Build history of the part. All positions in model axes, mm. Face numbers are marked on the shaded views. A direction names the side the tool comes from. Coordinates: 2 decimals unless noted, no trailing zeros. Order: outer loops, then holes, each group sorted by start corner. A loop starts at its lowest first (then second) coordinate and runs counter-clockwise, first axis right, second up. Notation, with made-up numbers: M 86,-35 L 118,-35 A35 cw 118,1 Z; hole C 27,8.5 d3. An arc over 180 degrees is marked long. Write item = value, one per line. Start each with the question number.
Q1. Pull direction X, two halves, no side cores. Call the marked faces 1, 2 and 3: released by +X, released by -X, zero draft, split by the parting line, or undercut.
Q2. Pin check, flat tips, straight feed: P1, Ø0.9, axis at y = -18.5, z = 9.5, coming from the +X side; P2, Ø2, axis at x = 0.5, y = -22.5, coming from the +Z side; P3, Ø0.5, axis at y = -9, z = 8.5, coming from the +X side; P4, Ø0.8, axis at x = -11, z = 8.5, coming from the +Y side. Stop position of each tip, or through.
Q3. Band-saw the part on D-D on x = -18. Write the cut outline in (y, z), plus the area to 3 significant figures.
Q4. 3-axis set-ups, long thin cutter, end or side, ignore diameter. For the marked faces 4, 5 and 6: which of +Z, -Z, +X, -X, +Y, -Y reach the whole face in a straight line?
Q5. Drill centre lines: probe 1 along X at (y, z) = (-17, 15); probe 2 along X at (y, z) = (-18.25, 9); probe 3 along X at (y, z) = (-24.25, 9). Where is each one in solid material? Low to high.
Q6. Band-saw the part on B-B on z = 14.75. Write the cut outline in (x, y), plus the area to 3 significant figures.
Q7. Band-saw the part on A-A on z = 10. Write the cut outline in (x, y), plus the area to 3 significant figures.
Q8. Band-saw the part on C-C on z = 7. State how many separate pieces and enclosed holes the cut face has, plus the area to 3 significant figures.
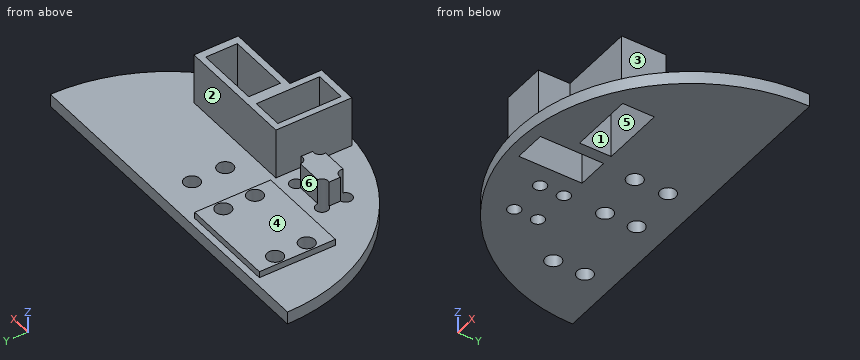
```python
from build123d import *

# Parameters (mm, degrees)
SKETCH009_W      = 5
SKETCH009_H      = 10
SKETCH009_W_2    = 10
SKETCH009_H_2    = 5
EXTRUDE008_DEPTH = 10
SKETCH008_R      = 1
EXTRUDE007_DEPTH = 6
SKETCH007_R      = 1.25
EXTRUDE006_DEPTH = 3
SKETCH004_R      = 1.25
EXTRUDE005_DEPTH = 3
SKETCH005_W      = 6.5
SKETCH005_H      = 4
EXTRUDE004_DEPTH = 4
SKETCH006_W      = 12
SKETCH006_H      = 7
SKETCH006_W_2    = 7
SKETCH006_H_2    = 12
EXTRUDE003_DEPTH = 8
SKETCH003_W      = 15
SKETCH003_H      = 12
EXTRUDE002_DEPTH = 1
EXTRUDE001_DEPTH = 6
EXTRUDE_DEPTH    = 8


with BuildPart() as usb_cuts:
    # Sketch009 → Extrude008 (new body)
    with BuildSketch(Plane.XY.offset(16)):
        with Locations((0, -20.5)):
            Rectangle(SKETCH009_W, SKETCH009_H)
        with Locations((9.25, -18)):
            Rectangle(SKETCH009_W_2, SKETCH009_H_2)
    extrude(amount=-EXTRUDE008_DEPTH)


with BuildPart() as reset_leads:
    # Sketch008 → Extrude007 (new body)
    with BuildSketch(Plane.XY.offset(12)):
        with Locations((-12, -16)):
            Circle(SKETCH008_R)
        with Locations((-6, -19.75)):
            Circle(SKETCH008_R)
        with Locations((-6, -16)):
            Circle(SKETCH008_R)
        with Locations((-12, -19.75)):
            Circle(SKETCH008_R)
    extrude(amount=-EXTRUDE007_DEPTH)


with BuildPart() as momentary_leads:
    # Sketch007 → Extrude006 (new body)
    with BuildSketch(Plane.XY.offset(9)):
        with Locations((-18, -9.5)):
            Circle(SKETCH007_R)
        with Locations((-18, -4.5)):
            Circle(SKETCH007_R)
        with Locations((-6, -9.5)):
            Circle(SKETCH007_R)
        with Locations((-6, -4.5)):
            Circle(SKETCH007_R)
    extrude(amount=-EXTRUDE006_DEPTH)


with BuildPart() as obj1:
    # Sketch004 → Extrude005 (new body)
    with BuildSketch(Plane.XY.offset(8)):
        with Locations((2, -10.25)):
            Circle(SKETCH004_R)
        with Locations((2, -5)):
            Circle(SKETCH004_R)
    extrude(amount=-EXTRUDE005_DEPTH)


with BuildPart() as obj2:
    # Sketch005 → Extrude004 (new body)
    with BuildSketch(Plane.XY.offset(8)):
        with Locations((-9, -18)):
            Rectangle(SKETCH005_W, SKETCH005_H)
    extrude(amount=EXTRUDE004_DEPTH)


with BuildPart() as usb_ports001:
    # Sketch006 → Extrude003 (new body)
    with BuildSketch(Plane.XY.offset(8)):
        with Locations((9.5, -18)):
            Rectangle(SKETCH006_W, SKETCH006_H)
        with Locations((0, -20.5)):
            Rectangle(SKETCH006_W_2, SKETCH006_H_2)
    extrude(amount=EXTRUDE003_DEPTH)


with BuildPart() as momentary_button:
    # Sketch003 → Extrude002 (new body)
    with BuildSketch(Plane.XY.offset(8)):
        with Locations((-12, -7)):
            Rectangle(SKETCH003_W, SKETCH003_H)
    extrude(amount=EXTRUDE002_DEPTH)


with BuildPart() as body_cut:
    # Sketch002 → Extrude001 (new body)
    with BuildSketch(Plane.XY):
        with BuildLine():
            ThreePointArc((-27.5, 0), (0, -27.5), (27.5, 0))
            Line((-27.5, 0), (27.5, 0))
        make_face()
    extrude(amount=EXTRUDE001_DEPTH)


with BuildPart() as cut004:
    # Sketch001 → Extrude (new body)
    with BuildSketch(Plane.XY):
        with BuildLine():
            ThreePointArc((-27.5, 0), (0, -27.5), (27.5, 0))
            Line((-27.5, 0), (27.5, 0))
        make_face()
    extrude(amount=EXTRUDE_DEPTH)

    # Cut: cut Body Cut
    add(body_cut.part, mode=Mode.SUBTRACT)

    # Fusion: union Momentary Button
    add(momentary_button.part)

    # Fusion001: union USB Ports001
    add(usb_ports001.part)

    # Fusion002: union obj2
    add(obj2.part)

    # Cut001: cut obj1
    add(obj1.part, mode=Mode.SUBTRACT)

    # Cut002: cut momentary Leads
    add(momentary_leads.part, mode=Mode.SUBTRACT)

    # Cut003: cut Reset Leads
    add(reset_leads.part, mode=Mode.SUBTRACT)

    # Cut004: cut USB Cuts
    add(usb_cuts.part, mode=Mode.SUBTRACT)


solid = cut004.part
```
Recorded:
q1.face_1 = undercut
q1.face_2 = zero draft
q1.face_3 = released by +X
q2.P1 = 15.5
q2.P2 = through
q2.P3 = -4.5
q2.P4 = -1
q3.outline = M -20.79,6 L -10.75,6 L -10.75,9 L -13,9 L -13,8 L -20.79,8 Z; M -8.25,6 L -5.75,6 L -5.75,9 L -8.25,9 Z; M -3.25,6 L 0,6 L 0,8 L -1,8 L -1,9 L -3.25,9 Z
q3.area = 38.6 mm2
q4.face_4 = +Z, +X, -X, +Y
q4.face_5 = +Z, -Z
q4.face_6 = +Z, -X
q5.probe_1 = -3.5 to -2.5, 2.5 to 4.25, 14.25 to 15.5
q5.probe_2 = -12.25 to -5.75, -3.5 to -2.5, 2.5 to 4.25, 14.25 to 15.5
q5.probe_3 = -3.5 to -2.5, 2.5 to 3.5
q6.outline = M -3.5,-26.5 L 3.5,-26.5 L 3.5,-21.5 L 15.5,-21.5 L 15.5,-14.5 L -3.5,-14.5 Z; hole M -2.5,-25.5 L 2.5,-25.5 L 2.5,-15.5 L -2.5,-15.5 Z; hole M 4.25,-20.5 L 14.25,-20.5 L 14.25,-15.5 L 4.25,-15.5 Z
q6.area = 68.0 mm2
q7.outline = M -12.25,-18.78 A1 cw -11.03,-20 L -6.97,-20 A1 cw -5.75,-18.78 L -5.75,-16.97 A1 cw -7,-16 L -11,-16 A1 cw -12.25,-16.97 Z; M -3.5,-26.5 L 3.5,-26.5 L 3.5,-21.5 L 15.5,-21.5 L 15.5,-14.5 L -3.5,-14.5 Z; hole M -2.5,-25.5 L 2.5,-25.5 L 2.5,-15.5 L -2.5,-15.5 Z; hole M 4.25,-20.5 L 14.25,-20.5 L 14.25,-15.5 L 4.25,-15.5 Z
q7.area = 89.2 mm2
q8.separate_pieces = 1
q8.enclosed_holes = 12
q8.area = 1,050 mm2
